Input: part model. Units: mm. Frame: model coordinates. Face numbers are marked on the shaded views. A direction names the side the tool comes from. Give positions to 0.01 mm unless a question says otherwise; leave off trailing zeros. Write each loop counter-clockwise with the first axis right and the second up, starting at its lowest first coordinate (ties: lowest second). Pieces come first, ordered by that corner, then holes. Notation, with made-up numbers: (2.25, 25) - (20.25, 25) arc R19 cw to (20.25, 32) - close; hole circle Ø4 at (57, -26.5). An arc over 180 degrees is marked (long way). Use a Markdown table: item, result. Add a question column.
1. Set-up query: the marked faces 5, 6, 7, 8 and 9. Return all of +Z, -Z, +X, -X, +Y, -Y with unobstructed straight access to the full face (end or side cutting, diameter ignored); none if empty.
2. Mould query, pull axis Y, two halves, no side actions, for the marked faces 1, 2, 3 and 4. Classes: released by +Y, released by -Y, zero draft, split by the parting line, or undercut.
3. Pin query (flat end, axial travel): pin 1 (6 mm diameter, centred on x = 31.5, y = 12.5, fed in from +Z); pin 2 (6.5 mm diameter, centred on x = 31, y = 53.69, fed in from -Z); pin 3 (19 mm diameter, centred on x = 25, y = -54.5, fed in from -Z). Return the tip coordinate at first contact, or that it passes through.
4. Section query B-B, the plane x = 62. Return loops of the section in (y, z), plus the area to 3 significant figures.
5. Section query A-A, the plane z = 16. Count the separate pieces of the cut face and the enclosed holes in it, plus the area to 3 significant figures.
6. Material intervals for probe 1 along Y at (x, z) = (-6, 4.75); probe 2 along Y at (x, z) = (0, 3); probe 3 along X at (y, z) = (5, 1.25), sorted ascending.
```python
from build123d import *

# Parameters (mm, degrees)
CUT_EXTRUDE15_DEPTH      = 97.415368098
CUT_EXTRUDE15_DEPTH_BACK = 97.415368098
SKETCH53_R               = 2.5
CUT_EXTRUDE16_DEPTH      = 93.391600197
SKETCH88_R               = 1.75
SKETCH88_R_2             = 2
CUT_EXTRUDE17_DEPTH      = 94.459768752


with BuildPart() as part:
    # Sketch51 → Revolve2 (revolve)
    with BuildSketch(Plane(origin=(0, 0, 0), x_dir=(0, 0, -1), z_dir=(1, 0, 0)), mode=Mode.PRIVATE) as revolve2_sk:
        Polygon((-13.54338235, 57.5), (0, 40.5), (0, 0), (-6, 0), (-6, 38.402164253), (-19.54338235, 55.402164253), (-19.54338235, 67.5), (-13.54338235, 67.5), align=None)
    revolve(revolve2_sk.sketch.rotate(Axis((0, 0, 0), (0, 0, -1)), 90), axis=Axis((0, 0, 0), (0, 0, -1)))

    # Sketch52 → Cut-Extrude15 (cut, two sides: drawn at the far end of the back side and taken through both)
    with BuildSketch(Plane(origin=(0, 0, 13.54338235), x_dir=(-1, 0, 0), z_dir=(0, 0, -1)).offset(-CUT_EXTRUDE15_DEPTH_BACK)):
        Polygon((-37.295847234, 71.348937003), (-6, 40.053089768), (6, 40.053089768), (37.295847234, 71.348937003), align=None)
        Polygon((31.68699324, 25.222697307), (37.68699324, 14.830392462), (80.437915594, 3.375317341), (43.14206836, 67.973619662), align=None)
        Polygon((37.68699324, -14.830392462), (31.68699324, -25.222697307), (43.14206836, -67.973619662), (80.437915594, -3.375317341), align=None)
        Polygon((6, -40.053089768), (-6, -40.053089768), (-37.295847234, -71.348937003), (37.295847234, -71.348937003), align=None)
        Polygon((-31.68699324, -25.222697307), (-37.68699324, -14.830392462), (-80.437915594, -3.375317341), (-43.14206836, -67.973619662), align=None)
        Polygon((-37.68699324, 14.830392462), (-31.68699324, 25.222697307), (-43.14206836, 67.973619662), (-80.437915594, 3.375317341), align=None)
    extrude(amount=CUT_EXTRUDE15_DEPTH + CUT_EXTRUDE15_DEPTH_BACK, mode=Mode.SUBTRACT)

    # Sketch53 → Cut-Extrude16 (cut, through all)
    with BuildSketch(Plane(origin=(0, 0, 13.54338235), x_dir=(-1, 0, 0), z_dir=(0, 0, -1))):
        with Locations((62, 0)):
            Circle(SKETCH53_R)
        with Locations((31, -53.693575035)):
            Circle(SKETCH53_R)
        with Locations((-31, -53.693575035)):
            Circle(SKETCH53_R)
        with Locations((-62, 0)):
            Circle(SKETCH53_R)
        with Locations((-31, 53.693575035)):
            Circle(SKETCH53_R)
        with Locations((31, 53.693575035)):
            Circle(SKETCH53_R)
    extrude(amount=-CUT_EXTRUDE16_DEPTH, mode=Mode.SUBTRACT)

    # Sketch88 → Cut-Extrude17 (cut, through all)
    with BuildSketch(Plane(origin=(0, 0, 0), x_dir=(-1, 0, 0), z_dir=(0, 0, -1))):
        with Locations((0, 12)):
            Circle(SKETCH88_R)
        with Locations((10.392304845, 6)):
            Circle(SKETCH88_R)
        with Locations((10.392304845, -6)):
            Circle(SKETCH88_R)
        with Locations((0, -12)):
            Circle(SKETCH88_R)
        with Locations((-10.392304845, -6)):
            Circle(SKETCH88_R)
        with Locations((-10.392304845, 6)):
            Circle(SKETCH88_R)
        with Locations((6, -10.392304845)):
            Circle(SKETCH88_R_2)
        with Locations((-12, 0)):
            Circle(SKETCH88_R_2)
        with Locations((6, 10.392304845)):
            Circle(SKETCH88_R_2)
    extrude(amount=-CUT_EXTRUDE17_DEPTH, mode=Mode.SUBTRACT)


solid = part.part
```
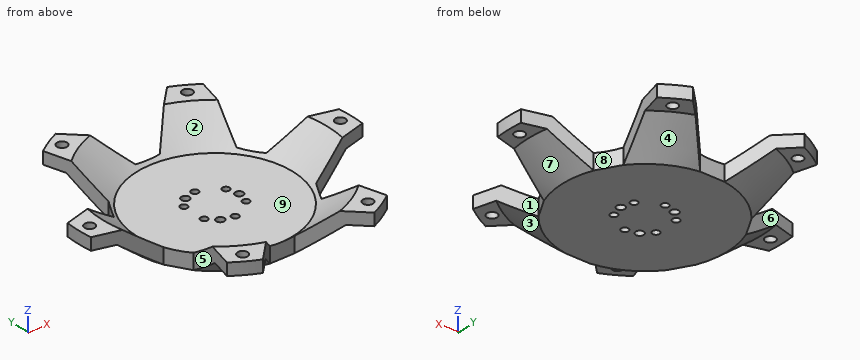
Result sheet:
| question | item | result |
|---|---|---|
| 1 | face 5 | +Z, -Z, -X |
| 1 | face 6 | +Z, -Z, -X, +Y |
| 1 | face 7 | -Z, +X |
| 1 | face 8 | +Z, -Z, +X |
| 1 | face 9 | +Z |
| 2 | face 1 | undercut |
| 2 | face 2 | undercut |
| 2 | face 3 | released by -Y |
| 2 | face 4 | released by +Y |
| 3 | pin 1 | stops at z = 6 |
| 3 | pin 2 | stops at z = 13.54 |
| 3 | pin 3 | stops at z = 7.94 |
| 4 | outline | (-8.32, 13.54) - (-2.5, 13.54) - (-2.5, 19.54) - (-8.32, 19.54) - close; (2.5, 13.54) - (8.32, 13.54) - (8.32, 19.54) - (2.5, 19.54) - close |
| 4 | area | 69.8 mm² |
| 5 | separate pieces | 6 |
| 5 | enclosed holes | 6 |
| 5 | area | 1,730 mm² |
| 6 | probe 1 | y = -40.05 to -12.39, -8.39 to 8.39, 12.39 to 40.05 |
| 6 | probe 2 | y = -40.05 to -13.75, -10.25 to 10.25, 13.75 to 40.05 |
| 6 | probe 3 | x = -41.77 to -11.83, -8.96 to 8.96, 11.83 to 41.77 |
